```python
from build123d import *

# Parameters (mm, degrees)
F1_DEPTH = 7.62
F2_R     = 2.54


# Not quite as in the source:
# - a feature names something its author has since deleted; it is built from what else it names


with BuildPart() as f1:
    # F0 (on Right) → F1 (new body)
    with BuildSketch(Plane.YZ):
        Polygon((-39.391245693, -75.0930126251), (-21.611245693, -75.0930126251), (-21.611245693, 86.1969873749), (-36.851245693, 86.1969873749), (-39.391245693, 86.1969873749), (-39.391245693, 79.8469873749), (-36.851245693, 79.8469873749), (-36.851245693, 82.3869873749), (-25.421245693, 82.3869873749), (-25.421245693, -71.2830126251), (-36.851245693, -71.2830126251), (-36.851245693, -68.7430126251), (-39.391245693, -68.7430126251), align=None)
    extrude(amount=F1_DEPTH)

    # F2
    f2_edges = [f1.edges().sort_by_distance(p)[0] for p in [
        (3.81, -21.611246, -75.093013),
        (3.81, -21.611246, 86.196987),
    ]]
    fillet(f2_edges, radius=F2_R)


solid = f1.part
```
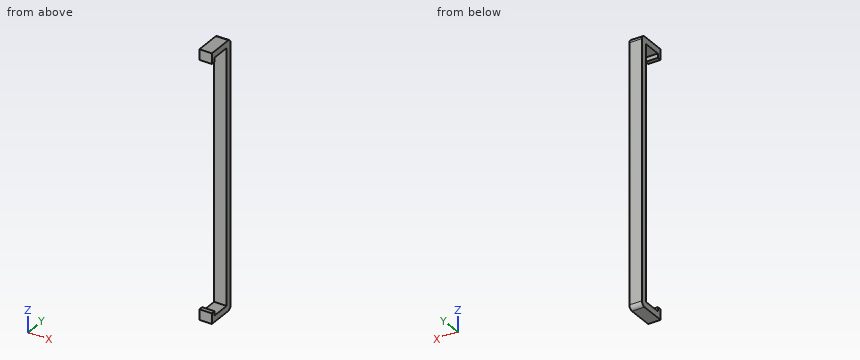
Input: part model. Units: mm. Frame: model coordinates. Coordinates: 2 decimals unless noted, no trailing zeros. Write each loop counter-clockwise with the first axis right and the second up, starting at its lowest first coordinate (ties: lowest second). Pieces come first, ordered by that corner, then holes. Notation, with made-up numbers: M -29.75,82.25 L 18.25,82.25 A13 cw 18.25,103.25 Z; hole C 78,-12.75 d6. An arc over 180 degrees is marked long. Use one line per item in the form item = value.
Q1. Material intervals for probe 1 along Z at (x, y) = (0.5, -37.75); probe 2 along Z at (x, y) = (1.5, -26.25); probe 3 along Y at (x, z) = (5.75, 45), sorted ascending. Write a range as from..to.
Answer below:
probe_1 = -75.09..-68.74, 79.85..86.2
probe_2 = -75.09..-71.28, 82.39..86.2
probe_3 = -25.42..-21.61
Q2. Section A-A (y = -31.25). Return loops of the section in (x, z), plus the area to 3 significant figures.
Answer below:
outline = M 0,-75.09 L 7.62,-75.09 L 7.62,-71.28 L 0,-71.28 Z; M 0,82.39 L 7.62,82.39 L 7.62,86.2 L 0,86.2 Z
area = 58.1 mm²
Q3. Section B-B (x = 1.25). Return loops of the section in (y, z).
Answer below:
outline = M -39.39,-75.09 L -24.15,-75.09 A2.54 ccw -21.61,-72.55 L -21.61,83.66 A2.54 ccw -24.15,86.2 L -39.39,86.2 L -39.39,79.85 L -36.85,79.85 L -36.85,82.39 L -25.42,82.39 L -25.42,-71.28 L -36.85,-71.28 L -36.85,-68.74 L -39.39,-68.74 Z
Q4. Section C-C (z = 69). Return loops of the section in (x, y).
Answer below:
outline = M 0,-25.42 L 7.62,-25.42 L 7.62,-21.61 L 0,-21.61 Z
Q5. First-contact query: pin 1 (1.5 mm diameter, centred on x = 3.5, z = 49.5, fed in from -Y); pin 2 (2 mm diameter, centred on y = -26.5, z = 1.5, fed in from +X). Flat tips, straight axial feed; report the tip coordinate or a pass-through.
Answer below:
pin_1 = -25.42
pin_2 = through
